```python
from build123d import *

# Parameters (mm, degrees)
F0_W      = 60
F0_H      = 50
F1_DEPTH  = 21
F2_W      = 58
F2_H      = 48
F3_DEPTH  = 20
F5_R      = 2
F6_R      = 4.5
F7_DEPTH  = 6
F10_W     = 11.5
F10_H     = 1
F11_DEPTH = 13
F12_W     = 2.5
F12_H     = 3.5
F13_DEPTH = 1
F14_R     = 4.5
F15_DEPTH = 1
F8_R      = 1.5
F16_DEPTH = 7
F9_R      = 1.5
F17_DEPTH = 7
F18_R     = 3.5
F18_R_2   = 1.5
F19_DEPTH = 1


with BuildPart() as f1:
    # F0 (on Top) → F1 (new body)
    with BuildSketch(Plane.XY):
        with Locations((-30, 25)):
            Rectangle(F0_W, F0_H)
    extrude(amount=F1_DEPTH)

    # F2 (on face) → F3 (cut)
    with BuildSketch(Plane.XY.offset(21)):
        with Locations((-30, 25)):
            Rectangle(F2_W, F2_H)
    extrude(amount=-F3_DEPTH, mode=Mode.SUBTRACT)

    # F5
    f5_edges = [f1.edges().sort_by_distance(p)[0] for p in [
        (-60, 50, 10.5),
        (0, 50, 10.5),
        (0, 0, 10.5),
        (-60, 0, 10.5),
    ]]
    fillet(f5_edges, radius=F5_R)

    # F6 (on face) → F7 (join)
    with BuildSketch(Plane.XY.offset(1)):
        with Locations((-22.1625890434, 6.5921834528)):
            Circle(F6_R)
        with Locations((-53.6625890434, 38.8921834528)):
            Circle(F6_R)
    extrude(amount=F7_DEPTH)

    # F10 (on face) → F11 (cut)
    with BuildSketch(Plane.XY.offset(21)):
        with Locations((-35.4789009094, 0.5)):
            Rectangle(F10_W, F10_H)
    extrude(amount=-F11_DEPTH, mode=Mode.SUBTRACT)

    # F12 (on face) → F13 (cut)
    with BuildSketch(Plane.XY.offset(1)):
        with Locations((-26.94821703, 11.3616460413)):
            Rectangle(F12_W, F12_H)
    extrude(amount=-F13_DEPTH, mode=Mode.SUBTRACT)

    # F14 (on face) → F15 (cut)
    with BuildSketch(Plane.XY.offset(1)):
        with Locations((-47.7578996122, 23)):
            Circle(F14_R)
    extrude(amount=-F15_DEPTH, mode=Mode.SUBTRACT)

    # F8 (on face) → F16 (cut)
    with BuildSketch(Plane.XY.offset(7)):
        with Locations((-53.6625890434, 38.8921834528)):
            Circle(F8_R)
    extrude(amount=-F16_DEPTH, mode=Mode.SUBTRACT)

    # F9 (on face) → F17 (cut)
    with BuildSketch(Plane.XY.offset(7)):
        with Locations((-22.1625890434, 6.5921834528)):
            Circle(F9_R)
    extrude(amount=-F17_DEPTH, mode=Mode.SUBTRACT)

    # F18 (on face) → F19 (cut)
    with BuildSketch(Plane(origin=(0, 0, 0), x_dir=(1, 0, 0), z_dir=(0, 0, -1))):
        with Locations((-22.1625890434, -6.5921834528)):
            Circle(F18_R)
        with Locations((-22.1625890434, -6.5921834528)):
            Circle(F18_R_2, mode=Mode.SUBTRACT)
        with Locations((-53.6625890434, -38.8921834528)):
            Circle(F18_R)
        with Locations((-53.6625890434, -38.8921834528)):
            Circle(F18_R_2, mode=Mode.SUBTRACT)
    extrude(amount=-F19_DEPTH, mode=Mode.SUBTRACT)


solid = f1.part
```
Read the model definition and answer for the solid it produces. Units are mm, in the model's axes. A direction names the side the tool comes from. Round coordinates to 2 decimals unless told otherwise and drop trailing zeros. Write each loop counter-clockwise with the first axis right and the second up, starting at its lowest first coordinate (ties: lowest second). Pieces come first, ordered by that corner, then holes. Notation, with made-up numbers: M -24,-13.5 L 4,-13.5 A21 ccw 4,14.5 Z; hole C -18.75,3.25 d11. An arc over 180 degrees is marked long. One line per item, written item: value.
Q1. Which of the six approach directions +Z, -Z, +X, -X, +Y, -Y give full straight-line access (tool end or side, diameter ignored) to faces 4 (the cylindrical face through (-0.6, 0.57, 10.65)), 5 (the flat face through (-20.66, 7.32, 1)), 6 (the flat face through (-55, 40, 7))?
Data:
face 4: +Z, -Z, +X, -Y
face 5: -Z
face 6: +Z
Q2. Find section D-D on y = 15.5. Write down the section's boundary in (x, z).
Data:
outline: M -60,0 L 0,0 L 0,21 L -1,21 L -1,1 L -59,1 L -59,21 L -60,21 Z
Q3. For a pull along Y with two mould halves and no side action, classify faces 1 (the flat face through (-30, 50, 10)), 2 (the flat face through (-43.5, 49.2, 21)), 3 (the cylindrical face through (-18.824, 5.541, 0.493)) as +Y half, -Y half, draft (parallel to the pull), parting line (faces both ways), or undercut.
Data:
face 1: +Y half
face 2: draft
face 3: undercut
Q4. Straight lines are drawn through the part: line 1 (X direction, y = 16, z = 5.5); line 2 (Y direction, x = -20, z = 10.75); line 3 (Z direction, x = -39, y = 43.5). For each, find the intervals that lie inside material, in ascending order. Write a range as [from, to].
Data:
line 1: [-60, -59], [-1, 0]
line 2: [0, 1], [49, 50]
line 3: [0, 1]
Q5. Find section C-C on z = 4.75. Write down the section's boundary in (x, y), plus the area to 3 significant figures.
Data:
outline: M -60,2 A2 ccw -58,0 L -2,0 A2 ccw 0,2 L 0,48 A2 ccw -2,50 L -58,50 A2 ccw -60,48 Z; C -53.66,38.89 d9; C -22.16,6.59 d9; hole M -59,1 L -1,1 L -1,49 L -59,49 Z; hole C -53.66,38.89 d3; hole C -22.16,6.59 d3
area: 326 mm2
Q6. Flat-ended cylindrical pins translate along their axes: pin 1 Ø0.8 at (y, z) = (0.5, 16.5) entering from -X; pin 2 Ø3 at (x, y) = (-51, 5.5) entering from +Z; pin 3 Ø8 at (x, y) = (-22.16, 6.59) entering from -Z; pin 4 Ø3.5 at (x, y) = (-22.5, 8) entering from -Z. Find the tip coordinate at first contact, or state that the pin passes through.
Data:
pin 1: x = -59.67
pin 2: z = 1
pin 3: z = 0
pin 4: z = 1
Q7. Find section B-B on x = -6.5. Write down the section's boundary in (y, z), plus the area to 3 significant figures.
Data:
outline: M 0,0 L 50,0 L 50,21 L 49,21 L 49,1 L 1,1 L 1,21 L 0,21 Z
area: 90.0 mm2
Q8. Find section A-A on y = 23. Write down the section's boundary in (x, z), plus the area to 3 significant figures.
Data:
outline: M -60,0 L -52.26,0 L -52.26,1 L -59,1 L -59,21 L -60,21 Z; M -43.26,0 L 0,0 L 0,21 L -1,21 L -1,1 L -43.26,1 Z
area: 91.0 mm2
